For this review, use the dimensioned drawing (mm, ordinates from the lowest corner) and the shaded views. Round coordinates to 2 decimals unless told otherwise and drop trailing zeros. Write each loop counter-clockwise with the first axis right and the second up, starting at its lowest first coordinate (ties: lowest second). Pieces come first, ordered by that corner, then holes. Notation, with made-up numbers: (8.25, -20) - (23.25, -20) arc R26 cw to (23.25, 13) - close; hole circle Ø3 at (41.25, 56.25). An arc over 180 degrees is marked (long way). Return JSON: item names as keys, results as strings.
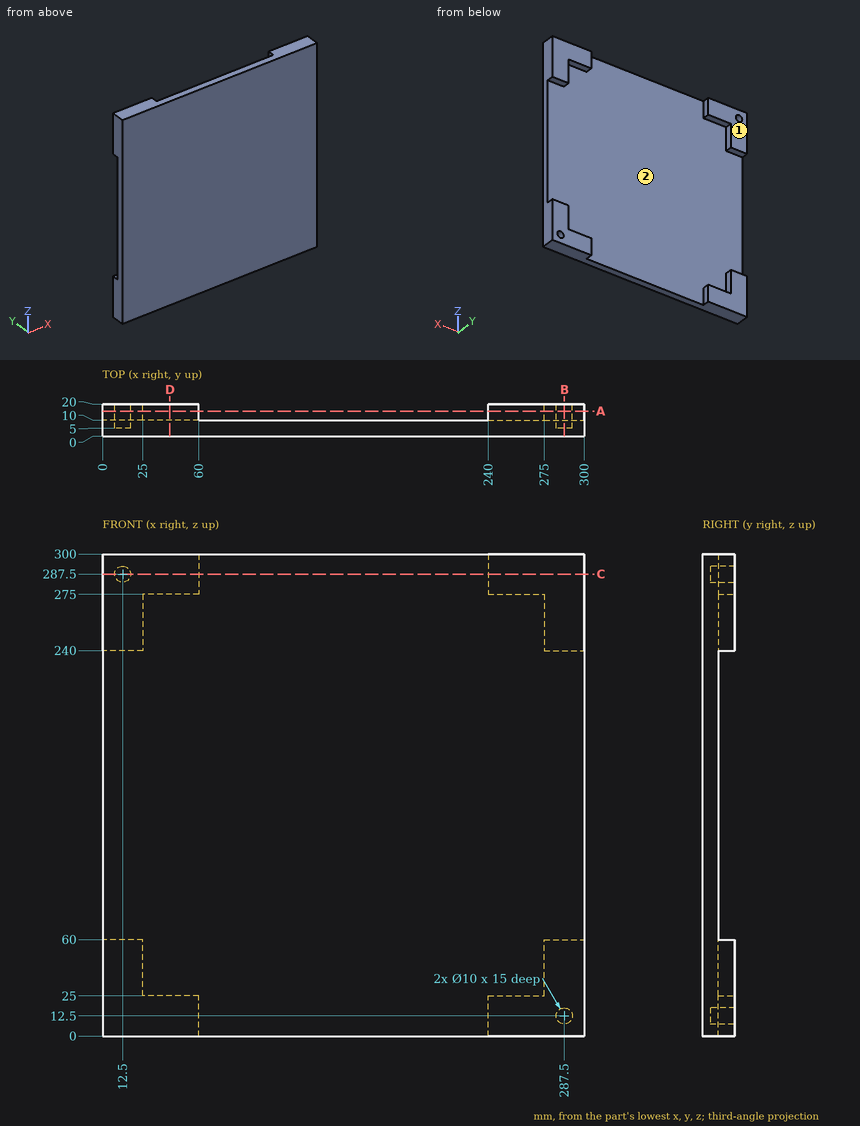
(1) Wall thickness on line 1 (X direction, y = 16.5, z = 287.5); line 2 (X direction, y = 14.25, z = 12.5); line 3 (Z direction, x = 246, y = 11): over which ranges is each line inside the solid? List them lowest first.
Filled in:
{"line 1": "x = 0 to 7.5, 17.5 to 60, 240 to 300", "line 2": "x = 0 to 60, 240 to 282.5, 292.5 to 300", "line 3": "z = 0 to 25, 275 to 300"}
(2) Add section D-D (x = 42). Write out the cut boundary in (y, z).
Filled in:
{"outline": "(0, 0) - (20, 0) - (20, 25) - (10, 25) - (10, 275) - (20, 275) - (20, 300) - (0, 300) - close"}
(3) Mouldability with a two-part tool opening along Z and no side actions: class the marked faces 1 and 2 as released by +Z, released by -Z, zero draft, split by the parting line, or undercut.
Filled in:
{"face 1": "zero draft", "face 2": "undercut"}
(4) Add section A-A (y = 15.5). Write out the cut boundary in (x, z), plus the area to 3 significant figures.
Filled in:
{"outline": "(0, 0) - (60, 0) - (60, 25) - (25, 25) - (25, 60) - (0, 60) - close; (0, 240) - (25, 240) - (25, 275) - (60, 275) - (60, 300) - (0, 300) - close; (240, 0) - (300, 0) - (300, 60) - (275, 60) - (275, 25) - (240, 25) - close; (240, 275) - (275, 275) - (275, 240) - (300, 240) - (300, 300) - (240, 300) - close; hole circle Ø10 at (12.5, 287.5); hole circle Ø10 at (287.5, 12.5)", "area": "9,340 mm2"}
(5) Add section C-C (z = 287.5). Write out the cut boundary in (x, y).
Filled in:
{"outline": "(0, 0) - (300, 0) - (300, 20) - (240, 20) - (240, 10) - (60, 10) - (60, 20) - (17.5, 20) - (17.5, 5) - (7.5, 5) - (7.5, 20) - (0, 20) - close"}
(6) Add section B-B (x = 287.5). Write out the cut boundary in (y, z).
Filled in:
{"outline": "(0, 0) - (20, 0) - (20, 7.5) - (5, 7.5) - (5, 17.5) - (20, 17.5) - (20, 60) - (10, 60) - (10, 240) - (20, 240) - (20, 300) - (0, 300) - close"}
(7) Clearance check with flat-ended pins moving along their axes: pin 1 Ø8 at (x, z) = (189, 224) entering from +Y; pin 2 Ø8 at (x, z) = (287.5, 12.5) entering from +Y. State where each tip first meets the part, or that it passes through.
Filled in:
{"pin 1": "stops at y = 10", "pin 2": "stops at y = 5"}
